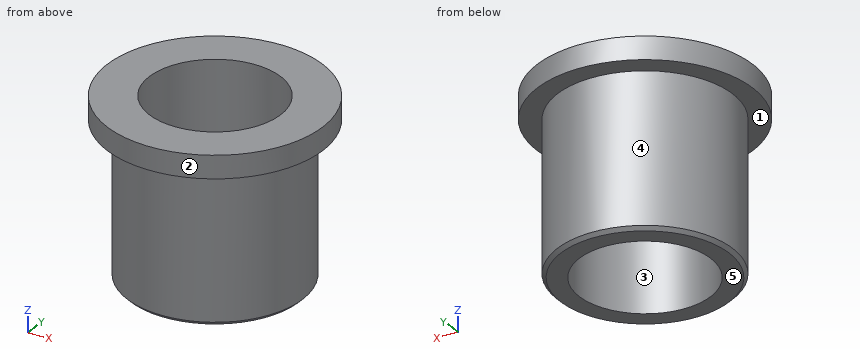
from build123d import *

# Parameters (mm, degrees)
F_1_4_0_75_DIAMETER_HOLE1_D = 19.05
CHAMFER1_SIZE               = 0.508


with BuildPart() as part:
    # Sketch1 → Revolve1 (revolve)
    with BuildSketch(Plane(origin=(0, 0, 0), x_dir=(0, 0, -1), z_dir=(1, 0, 0))):
        Polygon((0, 0), (-25.4, 0), (-25.4, 15.621), (-22.098, 15.621), (-22.098, 12.7), (0, 12.7), align=None)
    revolve(axis=Axis((0, 0, 0), (0, 0, -1)))

    # 1/4 (0.75) Diameter Hole1 (through all)
    with Locations(Plane.XY.offset(25.4)):
        with Locations((0, 0)):
            Hole(F_1_4_0_75_DIAMETER_HOLE1_D / 2)

    # Chamfer1
    chamfer1_edges = [part.edges().sort_by_distance(p)[0] for p in [
        (0, -12.7, 0),
    ]]
    chamfer(chamfer1_edges, length=CHAMFER1_SIZE)


solid = part.part
Model file for the job. Use its own axes, mm. Face numbers are marked on the shaded views. A direction names the side the tool comes from. Give positions to 0.01 mm unless a question says otherwise; leave off trailing zeros. Order: outer loops, then holes, each group sorted by start corner. A loop starts at its lowest first (then second) coordinate and runs counter-clockwise, first axis right, second up. Notation, with made-up numbers: M -29,-9 L -4,-9 A6 ccw -4,2 Z; hole C 72.5,-1 d11. An arc over 180 degrees is marked long. Write item = value, one per line.
Q1. Flat gauge pins, fed straight in: pin 1 (2 mm diameter, centred on x = -12, y = 7.5, fed in from -Z); pin 2 (2 mm diameter, centred on y = 2, z = 22.5, fed in from +X); pin 3 (12 mm diameter, centred on y = 2, z = 6, fed in from +X). Where does each tip first touch, or does it go through?
Derived:
pin_1 = 22.1
pin_2 = 15.59
pin_3 = 12.7
Q2. Tool access for the marked faces 1 and 2: list every direction of +Z, -Z, +X, -X, +Y, -Y with a clear straight run to the whole face (end or side of a thin tool).
Derived:
face_1 = -Z
face_2 = +Z, -Z
Q3. Cut at C-C, the plane z = 20.75. List the corners of the cut face in (x, y) (3 decimals), then the cut area to 3 significant figures.
Derived:
outline = C 0,0 d25.4; hole C 0,0 d19.05
area = 222 mm2
Q4. Two-plate mould, pull along X, no slides. Class the marked faces 3, 4 and 5: pulls with the +X half, pulls with the -X half, needs draft (parallel to the pull), parting line crosses it, or undercut.
Derived:
face_3 = undercut
face_4 = parting line crosses it
face_5 = needs draft
Q5. Drill centre lines: line 1 (Y direction, x = -6.5, z = 1); line 2 (X direction, y = 1, z = 7.25); line 3 (X direction, y = 7.5, z = 15.75). Where is each one in solid material? Low to high. Write a range as [from, to].
Derived:
line_1 = [-10.91, -6.96], [6.96, 10.91]
line_2 = [-12.66, -9.47], [9.47, 12.66]
line_3 = [-10.25, -5.87], [5.87, 10.25]
Q6. Cut at A-A, the plane y = 0. List the corners of the cut face in (x, z) (3 decimals).
Derived:
outline = M -15.621,22.098 L -12.7,22.098 L -12.7,0.508 L -12.192,0 L -9.525,0 L -9.525,25.4 L -15.621,25.4 Z; M 9.525,0 L 12.192,0 L 12.7,0.508 L 12.7,22.098 L 15.621,22.098 L 15.621,25.4 L 9.525,25.4 Z
